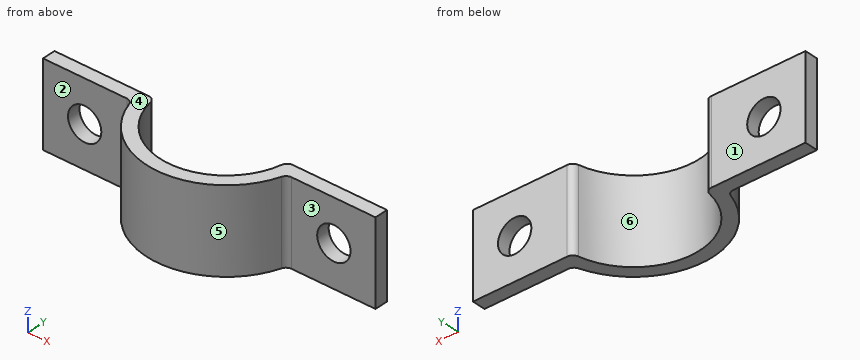
from build123d import *

# Parameters (mm, degrees)
BOSS_EXTRUDE2_DEPTH = 12.5
CUT_EXTRUDE1_REACH  = 13
SKETCH4_R           = 2.5


with BuildPart() as part:
    # Sketch3 → Boss-Extrude2 (new body)
    with BuildSketch(Plane.XY):
        with BuildLine():
            Line((-10.816653826, 19.01731952), (-19.949874371, 19.01731952))
            Line((-19.949874371, 19.01731952), (-24.949874371, 19.01731952))
            Line((-24.949874371, 19.01731952), (-24.949874371, 17.01731952))
            Line((-24.949874371, 17.01731952), (-19.949874371, 17.01731952))
            Line((-19.949874371, 17.01731952), (-12.369316877, 17.01731952))
            ThreePointArc((-12.369316877, 17.01731952), (-11.780968471, 16.82592706), (-11.417830963, 16.325011828))
            ThreePointArc((-11.417830963, 16.325011828), (0, 8.01731952), (11.417830963, 16.325011828))
            ThreePointArc((11.417830963, 16.325011828), (11.780968471, 16.82592706), (12.369316877, 17.01731952))
            Line((12.369316877, 17.01731952), (19.949874371, 17.01731952))
            Line((19.949874371, 17.01731952), (24.949874371, 17.01731952))
            Line((24.949874371, 17.01731952), (24.949874371, 19.01731952))
            Line((24.949874371, 19.01731952), (19.949874371, 19.01731952))
            Line((19.949874371, 19.01731952), (10.816653826, 19.01731952))
            ThreePointArc((10.816653826, 19.01731952), (10.177051677, 18.786025635), (9.83332166, 18.199137702))
            ThreePointArc((9.83332166, 18.199137702), (0, 10.01731952), (-9.83332166, 18.199137702))
            ThreePointArc((-9.83332166, 18.199137702), (-10.177051677, 18.786025635), (-10.816653826, 19.01731952))
        make_face()
    extrude(amount=BOSS_EXTRUDE2_DEPTH)

    # Sketch4 → Cut-Extrude1 (cut, up to next)
    with BuildSketch(Plane(origin=(0, 19.01731952, 0), x_dir=(1, 0, 0), z_dir=(0, 1, 0)), mode=Mode.PRIVATE) as cut_extrude1_sk1:
        with Locations((-18.699874371, -6.25)):
            Circle(SKETCH4_R)
    cut_extrude1_tool1 = extrude(cut_extrude1_sk1.sketch, amount=-CUT_EXTRUDE1_REACH, mode=Mode.PRIVATE) & part.part
    add(cut_extrude1_tool1.solids().sort_by_distance((-18.699874, 19.01732, 6.25))[0], mode=Mode.SUBTRACT)
    # Sketch4 → Cut-Extrude1 (cut, up to next)
    with BuildSketch(Plane(origin=(0, 19.01731952, 0), x_dir=(1, 0, 0), z_dir=(0, 1, 0)), mode=Mode.PRIVATE) as cut_extrude1_sk2:
        with Locations((18.699874371, -6.25)):
            Circle(SKETCH4_R)
    cut_extrude1_tool2 = extrude(cut_extrude1_sk2.sketch, amount=-CUT_EXTRUDE1_REACH, mode=Mode.PRIVATE) & part.part
    add(cut_extrude1_tool2.solids().sort_by_distance((18.699874, 19.01732, 6.25))[0], mode=Mode.SUBTRACT)


solid = part.part
Can you work these out from the model? Positions are in its coordinate system, mm. Face numbers are marked on the shaded views. A direction names the side the tool comes from. Give positions to 0.01 mm unless a question says otherwise; leave off trailing zeros. Loops run counter-clockwise (first coordinate to the right, second up) from the corner with the lowest first, then second, coordinate; pieces in that order, holes last. Notation, with made-up numbers: (-39, -32.75) - (-12, -32.75) arc R31 cw to (-12, -4.75) - close; hole circle Ø9 at (78.5, 89). An arc over 180 degrees is marked (long way). Return JSON: item names as keys, results as strings.
1. We'd pull the mould along X, two halves only. Please class the marked faces 4, 5 and 6: +X half, -X half, draft (parallel to the pull), parting line (faces both ways), or undercut.
Output values:
{"face 4": "draft", "face 5": "parting line", "face 6": "undercut"}
2. I want a section at A-A on z = 6.25. Please give me the cut outline in (x, y).
Output values:
{"outline": "(-24.95, 17.02) - (-21.2, 17.02) - (-21.2, 19.02) - (-24.95, 19.02) - close; (-16.2, 17.02) - (-12.37, 17.02) arc R1 cw to (-11.42, 16.33) arc R12 ccw to (11.42, 16.33) arc R1 cw to (12.37, 17.02) - (16.2, 17.02) - (16.2, 19.02) - (10.82, 19.02) arc R1 ccw to (9.83, 18.2) arc R10 cw to (-9.83, 18.2) arc R1 ccw to (-10.82, 19.02) - (-16.2, 19.02) - close; (21.2, 17.02) - (24.95, 17.02) - (24.95, 19.02) - (21.2, 19.02) - close"}
3. I want a section at D-D on x = -19. Please give me the cut outline in (y, z).
Output values:
{"outline": "(17.02, 0) - (19.02, 0) - (19.02, 3.77) - (17.02, 3.77) - close; (17.02, 8.73) - (19.02, 8.73) - (19.02, 12.5) - (17.02, 12.5) - close"}
4. I want a section at C-C on z = 1.25. Please give me the cut outline in (x, y), and give its area (3 significant figures).
Output values:
{"outline": "(-24.95, 17.02) - (-12.37, 17.02) arc R1 cw to (-11.42, 16.33) arc R12 ccw to (11.42, 16.33) arc R1 cw to (12.37, 17.02) - (24.95, 17.02) - (24.95, 19.02) - (10.82, 19.02) arc R1 ccw to (9.83, 18.2) arc R10 cw to (-9.83, 18.2) arc R1 ccw to (-10.82, 19.02) - (-24.95, 19.02) - close", "area": "118 mm²"}
5. I'm going to push flat-ended pins straight in: pin 1 Ø5 at (x, z) = (3.5, 6) entering from +Y; pin 2 Ø6 at (x, z) = (-16.5, 3.5) entering from -Y; pin 3 Ø6 at (y, z) = (9.5, 5) entering from +X; pin 4 Ø4 at (x, z) = (18.7, 6.25) entering from +Y. Where does each tip first touch, or does it pass through?
Output values:
{"pin 1": "stops at y = 12.02", "pin 2": "stops at y = 17.02", "pin 3": "stops at x = 9.35", "pin 4": "passes through"}
6. I want a section at B-B on y = 10.5. Please give me the cut outline in (x, z), and give its area (3 significant figures).
Output values:
{"outline": "(-7.31, 0) - (-3.07, 0) - (-3.07, 12.5) - (-7.31, 12.5) - close; (3.07, 0) - (7.31, 0) - (7.31, 12.5) - (3.07, 12.5) - close", "area": "106 mm²"}
7. For the marked faces 1, 2 and 3, which set-ups out of +Z, -Z, +X, -X, +Y, -Y let a thin tool reach every point of the face, with its end or its side?
Output values:
{"face 1": "+Z, -Z, +X, -X, +Y", "face 2": "+Z, -Z, -X, -Y", "face 3": "+Z, -Z, +X, -Y"}
8. If I drill on line 1 (X direction, y = 18.6, z = 6.25); line 2 (X direction, y = 17.85, z = 6.25); line 3 (Y direction, x = 21, z = 1.25), over which ranges is the centre line in solid material (lowest first)?
Output values:
{"line 1": "x = -24.95 to -21.2, -16.2 to -10, 10 to 16.2, 21.2 to 24.95", "line 2": "x = -24.95 to -21.2, -16.2 to -9.76, 9.76 to 16.2, 21.2 to 24.95", "line 3": "y = 17.02 to 19.02"}
